Autodesk Inventor part; units mm, degrees
ref_plane "YZ Plane" through (0, 0, 0) normal (1, 0, 0) x (0, 1, 0)
ref_plane "XZ Plane" through (0, 0, 0) normal (0, 1, 0) x (-1, 0, 0)
ref_plane "XY Plane" through (0, 0, 0) normal (0, 0, 1) x (1, 0, 0)
sketch "Sketch1" plane through (0, 0, 0) normal (0, 0, 1) x (1, 0, 0)
  circle A0 centre (0, 0) radius 3.175
  dimension "d0" = 6.35
extrude "Extrusion1" add sketch "Sketch1" along normal mid plane 259
sketch "Sketch2" plane through (0, 0, 0) normal (0, 1, 0) x (-1, 0, 0)
  circle A0 centre (0, 129.875) radius 6.35
  circle A1 centre (0, -129.875) radius 6.35
  line L0 (-3.175, -129.5) -> (-3.175, 129.5)
  line L1 (-3.175, 0) -> (16.7407, 0)
  point P0 (3.175, -105.625)
  dimension "d4" = 259.75
  dimension "d5" = 129.875
  dimension "d6" = 12.7
  dimension "d7" = 12.7
extrude "Extrusion2" add sketch "Sketch2" along normal blind 10 and the other way blind 3.175
sketch "Sketch3" plane through (0, 10, 129.875) normal (0, 1, 0) x (1, 0, 0)
  circle A0 centre (0, 0) radius 6.35
  circle A1 centre (0, 259.75) radius 6.35
  point P0 (0, 129.875)
hole "Hole1" at (0, 10, 129.875) at (0, 10, -129.875) direction (0, -1, 0) diameter 2.1565 end through all
sketch "Sketch9" plane through (0, -3.175, 129.875) normal (0, -1, 0) x (1, 0, 0)
  line L0 (-3.45, 3.1) -> (3.45, 3.1)
  line L1 (3.45, 3.1) -> (3.45, -3.1)
  line L2 (3.45, -3.1) -> (-3.45, -3.1)
  line L3 (-3.45, -3.1) -> (-3.45, 3.1)
  line L4 (-3.45, 3.1) -> (3.45, -3.1) construction
  line L5 (3.45, 3.1) -> (-3.45, -3.1) construction
  line L6 (0, -129.875) -> (-12.946, -129.875)
  line L7 (-3.45, -262.85) -> (3.45, -262.85)
  line L8 (3.45, -262.85) -> (3.45, -256.65)
  line L9 (3.45, -256.65) -> (-3.45, -256.65)
  line L10 (-3.45, -256.65) -> (-3.45, -262.85)
  point P0 (0, 0)
  dimension "d28" = 6.9
  dimension "d29" = 6.2
extrude "Extrusion6" cut sketch "Sketch9" against normal blind 3
properties part number "Solar_Panel_Bar"
Here's how the part is built. I have some questions about the finished solid (model axes, mm). A direction names the side the tool comes from. Coordinates: 2 decimals unless noted, no trailing zeros. Write each loop counter-clockwise with the first axis right and the second up, starting at its lowest first coordinate (ties: lowest second). Pieces come first, ordered by that corner, then holes.
1) I'm going to push flat-ended pins straight in: pin 1 (3 mm diameter, centred on x = 1.5, z = 129, fed in from -Y) (3 decimals); pin 2 (6 mm diameter, centred on x = -1, z = 98.5, fed in from +Y) (3 decimals); pin 3 (1 mm diameter, centred on y = 2.5, z = 46, fed in from -X). Where does each tip first touch, or does it pass through?
Filled in:
pin 1: stops at y = -0.175
pin 2: stops at y = 3.175
pin 3: stops at x = -2.47
2) Which directions (+Z, -Z, +X, -X, +Y, -Y) give clear straight access to the entire face, cutting with the end or side of a thin tool? Please do faces 1 (the face through (-1, -0.175, 131)), 2 (the face through (-0.69, 3.1, -1.74)), 3 (the face through (0, -3.175, -134)).
Filled in:
face 1: -Y
face 2: none
face 3: +Z, -Z, +X, -X, -Y
3) If we section it at B-B (y = 6.5): Count the separate pieces of the cut face and the enclosed holes in it, plus the area to 3 significant figures.
Filled in:
separate pieces: 2
enclosed holes: 2
area: 246 mm2
4) Thinking about a two-plate mould opening in Z: for faces 4 (the face through (1.377, 3.505, -136.074)), 5 (the face through (0.1, 10, -131.2)), which applies, +Z half, -Z half, draft (parallel to the pull), parting line (faces both ways), or undercut?
Filled in:
face 4: undercut
face 5: draft
5) If we section it at A-A (z = -43): List the corners of the cut face in (x, y) for me (3 decimals).
Filled in:
outline: circle Ø6.35 at (0, 0)
6) If I drill on line 1 (Z direction, x = 0, y = 7) (3 decimals); line 2 (Z direction, x = 0, y = 2) (3 decimals); line 3 (X direction, y = -0.5, z = -120), over which ranges is the centre line in solid material (lowest first)?
Filled in:
line 1: z = -136.225 to -130.953, -128.797 to -123.525, 123.525 to 128.797, 130.953 to 136.225
line 2: z = -136.225 to -130.953, -128.797 to 128.797, 130.953 to 136.225
line 3: x = -3.14 to 3.14
